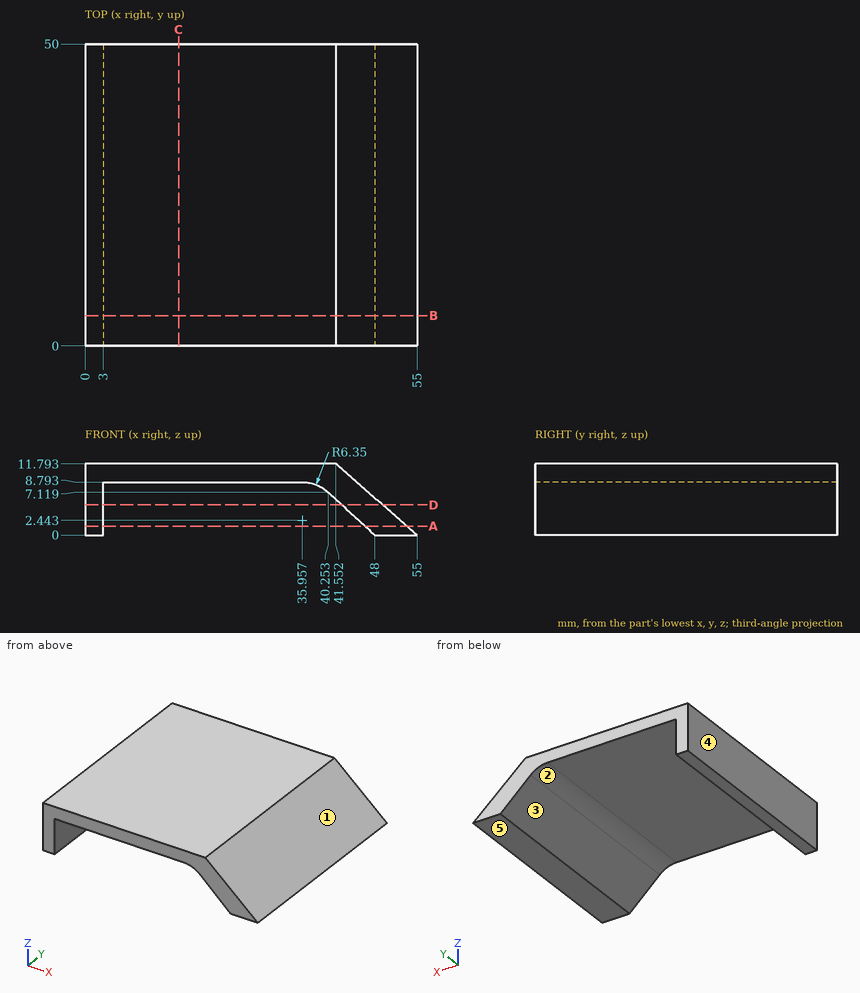
Check sheet for the drawn part. Datum: minimum x, y, z corner. Units: mm. A direction names the side the tool comes from. Round coordinates to 2 decimals unless told otherwise and drop trailing zeros. Order: outer loops, then holes, each group sorted by start corner. A loop starts at its lowest first (then second) coordinate and runs counter-clockwise, first axis right, second up.
1) Tool access check on the marked faces 1 and 2. Record the directions out of +Z, -Z, +X, -X, +Y, -Y that give a thin tool (end or side, any length) a straight path to the whole face; none if there is none.
2) Section check C-C (x = 15.5). Record the boundary of the cut face in (y, z), and give its area (3 significant figures).
3) Scan lines: line 1 (Z direction, x = 8.5, y = 18); line 2 (X direction, y = 29.5, z = 4.75) (1 decimal); line 3 (X direction, y = 25, z = 2.5). Record each from-to range of solid material in increasing order.
4) Section check D-D (z = 5). Record the boundary of the cut face in (x, y).
5) Section check B-B (y = 5). Record the boundary of the cut face in (x, z).
6) Section check A-A (z = 1.5). Record the boundary of the cut face in (x, y).
7) Mould release check, pull along X, two halves, no side actions. Record for the marked faces 3, 4 and 5: +X half, -X half, draft (parallel to the pull), parting line (faces both ways), or undercut.
8) Go/stop test with flat-tipped pins: pin 1 Ø1.5 at (x, z) = (20, 10) entering from -Y; pin 2 Ø4.5 at (y, z) = (13, 5) entering from +X (1 decimal); pin 3 Ø3 at (y, z) = (35.5, 5.5) entering from +X; pin 4 Ø3 at (x, z) = (13, 6.5) entering from +Y. Record where each tip stops, or that it passes through.
Result:
1. face 1: +Z, +X, +Y, -Y
1. face 2: -Z, +Y, -Y
2. outline: (0, 8.79) - (50, 8.79) - (50, 11.79) - (0, 11.79) - close
2. area: 150 mm2
3. line 1: z = 8.79 to 11.79
3. line 2: x = 0 to 3, 42.8 to 49.6
3. line 3: x = 0 to 3, 45.28 to 52.15
4. outline: (0, 0) - (3, 0) - (3, 50) - (0, 50) - close; (42.56, 0) - (49.3, 0) - (49.3, 50) - (42.56, 50) - close
5. outline: (0, 0) - (3, 0) - (3, 8.79) - (35.96, 8.79) arc R6.35 cw to (40.25, 7.12) - (48, 0) - (55, 0) - (41.55, 11.79) - (0, 11.79) - close
6. outline: (0, 0) - (3, 0) - (3, 50) - (0, 50) - close; (46.37, 0) - (53.29, 0) - (53.29, 50) - (46.37, 50) - close
7. face 3: undercut
7. face 4: -X half
7. face 5: draft
8. pin 1: stops at y = 0
8. pin 2: stops at x = 51.9
8. pin 3: stops at x = 50.44
8. pin 4: passes through
